Geometry: final body of the model. Coordinates: model frame, mm. A direction names the side the tool comes from. Give positions to 0.01 mm unless a question says otherwise; leave off trailing zeros. Loops run counter-clockwise (first coordinate to the right, second up) from the corner with the lowest first, then second, coordinate; pieces in that order, holes last. Notation, with made-up numbers: (24.25, 29) -> (49.25, 29) arc R17 ccw to (49.25, 44) -> close; hole circle Ø7 at (32, -9.5). An arc over 180 degrees is marked (long way). Answer in a Markdown table with one row per item. Add a question column.
1) Line query: line 1 (Y direction, x = -25, z = 1.05) (3 decimals); line 2 (Y direction, x = -19.05, z = 3.7); line 3 (Y direction, x = -10, z = 1.05). Output: solid intervals per line, ascending. Write a range as from..to.
2) Access query for faces 5 (the flat face through (-5, -15.24, 2)), 6 (the flat face through (0, -36, 2)). Directions: +Z, -Z, +X, -X, +Y, -Y. A direction counts if a zero-diameter tool reaches every point of the face in a straight line with its end or side. Return the directions, or none.
3) Section query C-C (x = -19.05). Return the cut outline in (y, z).
4) Section query A-A (x = -25). Give the number of separate pieces and of enclosed holes in the cut face, plus the area to 3 significant figures.
5) Section query B-B (y = -25). Return the cut outline in (x, z) (1 decimal).
6) Draft query along Y for faces 1 (the flat face through (-19, 38.1, 2)), 2 (the flat face through (-38.1, -10, 2)), 3 (the cylindrical face through (-15.27, -41.55, 2.35)), 4 (the flat face through (-10.16, 0, 2)). Return one class per face: +Y half, -Y half, draft (parallel to the pull), parting line (faces both ways), or undercut.
```python
from build123d import *

# Parameters (mm, degrees)
SKETCH2_W           = 38.1
SKETCH2_H           = 95.25
BOSS_EXTRUDE1_DEPTH = 4.7625
SKETCH3_R           = 2.125
SKETCH3_R_2         = 4.7625
SKETCH3_W           = 10.16
SKETCH3_H           = 30.48
CUT_EXTRUDE3_DEPTH  = 69.850663804


with BuildPart() as part:
    # Sketch2 → Boss-Extrude1 (new body)
    with BuildSketch(Plane.XY):
        with Locations((-19.05, -9.525)):
            Rectangle(SKETCH2_W, SKETCH2_H)
    extrude(amount=BOSS_EXTRUDE1_DEPTH)

    # Sketch3 → Cut-Extrude3 (cut, through all)
    with BuildSketch(Plane.XY):
        with Locations(Location((-25, 25, 0), (0, 0, 180))):
            Circle(SKETCH3_R)
        with Locations((25, 25)):
            Circle(SKETCH3_R)
        with Locations((25, -25)):
            Circle(SKETCH3_R)
        with Locations(Location((-25, -25, 0), (0, 0, 180))):
            Circle(SKETCH3_R)
        with Locations(Location((-19.05, -44.45, 0), (0, 0, 180))):
            Circle(SKETCH3_R_2)
        with Locations((-5.08, 0)):
            Rectangle(SKETCH3_W, SKETCH3_H)
    extrude(amount=CUT_EXTRUDE3_DEPTH, mode=Mode.SUBTRACT)


solid = part.part
```
Evaluation:
| question | item | result |
|---|---|---|
| 1 | line 1 | -57.15..-27.125, -22.875..22.875, 27.125..38.1 |
| 1 | line 2 | -57.15..-49.21, -39.69..38.1 |
| 1 | line 3 | -57.15..-15.24, 15.24..38.1 |
| 2 | face 5 | +Z, -Z, +X |
| 2 | face 6 | +Z, -Z, +X, +Y, -Y |
| 3 | outline | (-57.15, 0) -> (-49.21, 0) -> (-49.21, 4.76) -> (-57.15, 4.76) -> close; (-39.69, 0) -> (38.1, 0) -> (38.1, 4.76) -> (-39.69, 4.76) -> close |
| 4 | separate pieces | 3 |
| 4 | enclosed holes | 0 |
| 4 | area | 413 mm² |
| 5 | outline | (-38.1, 0) -> (-27.1, 0) -> (-27.1, 4.8) -> (-38.1, 4.8) -> close; (-22.9, 0) -> (0, 0) -> (0, 4.8) -> (-22.9, 4.8) -> close |
| 6 | face 1 | +Y half |
| 6 | face 2 | draft |
| 6 | face 3 | undercut |
| 6 | face 4 | undercut |
